```python
from build123d import *

# Parameters (mm, degrees)
SALIENTE_EXTRUIR1_DEPTH = 1.5
CROQUIS2_R              = 2.5
CROQUIS2_W              = 2.8
CROQUIS2_H              = 20
CORTAR_EXTRUIR1_DEPTH   = 11
CROQUIS4_W              = 2.8
CROQUIS4_H              = 25
CORTAR_EXTRUIR3_DEPTH   = 13
CROQUIS5_W              = 3
CROQUIS5_H              = 144.0002072
SALIENTE_EXTRUIR2_DEPTH = 15
CROQUIS6_R              = 4.1
CORTAR_EXTRUIR4_DEPTH   = 15
CROQUIS7_W              = 20.699997517
CROQUIS7_H              = 3
SALIENTE_EXTRUIR3_DEPTH = 3
CROQUIS8_W              = 20.699997553
CROQUIS8_H              = 3
SALIENTE_EXTRUIR4_DEPTH = 3


with BuildPart() as part:
    # Croquis1 → Saliente-Extruir1 (new, symmetric)
    with BuildSketch(Plane.XY):
        Polygon((419.401663173, 248.637154823), (419.401663173, 255.63715478), (422.401663173, 255.63715478), (422.401663173, 265.637154778), (419.401663173, 265.637154778), (419.401663173, 275.637154776), (422.401663173, 275.637154776), (422.401663173, 289.074445387), (426.151314195, 289.074445387), (426.151314195, 286.574445387), (429.151663171, 286.574445387), (429.151663171, 289.074445387), (431.101663171, 289.074445387), (431.101663171, 292.074445386), (429.151663171, 292.074445386), (429.151663171, 294.574864158), (426.151314195, 294.574864158), (426.151314195, 292.074445386), (422.401663173, 292.074445386), (422.401663173, 305.512154769), (419.401663173, 305.512154769), (419.401663173, 315.762154767), (422.401663173, 315.762154767), (422.401663173, 325.512154765), (419.401663173, 325.512154765), (419.401663173, 335.762154763), (422.401663173, 335.762154763), (422.401663173, 349.199445374), (426.151314195, 349.199445374), (426.151314195, 346.699445374), (429.151663171, 346.699445374), (429.151663171, 349.199445374), (431.101663171, 349.199445374), (431.101663171, 352.199445373), (429.151663171, 352.199445373), (429.151663171, 354.699864145), (426.151314195, 354.699864145), (426.151314195, 352.199445373), (422.401663173, 352.199445373), (422.401663173, 365.637154757), (419.401663173, 365.637154757), (419.401663173, 375.637154754), (422.401663173, 375.637154754), (422.401663173, 385.637154752), (419.401663173, 385.637154752), (419.401663173, 392.637154709), (431.9403463, 392.637154709), (431.9403463, 395.637154751), (444.561007671, 395.637160103), (444.561007671, 392.637160018), (453.092348422, 392.637160018), (453.092348422, 395.637160018), (462.04234842, 395.637160018), (462.04234842, 392.637192956), (464.82199969, 392.637192956), (464.82199969, 388.887541933), (462.321999691, 388.887541933), (462.321999691, 385.887192957), (464.82199969, 385.887192957), (464.82199969, 384.912192957), (467.82199969, 384.912192957), (467.82199969, 385.887192957), (470.322418461, 385.887192957), (470.322418461, 388.887541933), (467.82199969, 388.887541933), (467.82199969, 392.637192956), (470.601650959, 392.637192956), (470.601650959, 395.637192955), (479.551650957, 395.637192955), (479.551650957, 392.637269969), (488.101650956, 392.637269969), (488.101650956, 395.637269968), (500.701660095, 395.637269968), (500.701660095, 392.637258366), (519.401657648, 392.637258366), (519.401657648, 248.637051166), (500.701660131, 248.637051166), (500.701660131, 245.637039564), (488.101650991, 245.637039564), (488.101650991, 248.637039563), (479.551650993, 248.637039563), (479.551650993, 245.637116577), (470.601650995, 245.637116577), (470.601650995, 248.637116576), (467.821999725, 248.637116576), (467.821999725, 252.386767599), (470.322418497, 252.386767599), (470.322418497, 255.387116575), (467.821999725, 255.387116575), (467.821999725, 256.362116575), (464.821999726, 256.362116575), (464.821999726, 255.387116575), (462.321999727, 255.387116575), (462.321999727, 252.386767599), (464.821999726, 252.386767599), (464.821999726, 248.637116576), (462.042348456, 248.637116576), (462.042348456, 245.637149514), (453.092348458, 245.637149514), (453.092348458, 248.637149514), (444.561007707, 248.637149514), (444.561007707, 245.63714943), (431.940346335, 245.637154782), (431.940346335, 248.637154823), align=None)
    extrude(amount=SALIENTE_EXTRUIR1_DEPTH, both=True)

    # Croquis2 → Cortar-Extruir1 (cut)
    with BuildSketch(Plane.XY.offset(1.5)):
        with Locations((437.401663173, 340.137154766)):
            Circle(CROQUIS2_R)
        with Locations((437.401663173, 301.137154766)):
            Circle(CROQUIS2_R)
        with Locations((481.801663173, 320.637154766)):
            Rectangle(CROQUIS2_W, CROQUIS2_H)
        with Locations((456.001663173, 320.637154766)):
            Rectangle(CROQUIS2_W, CROQUIS2_H)
    extrude(amount=-CORTAR_EXTRUIR1_DEPTH, mode=Mode.SUBTRACT)

    # Croquis4 → Cortar-Extruir3 (cut)
    with BuildSketch(Plane(origin=(0, 0, -1.5), x_dir=(-1, 0, 0), z_dir=(0, 0, -1))):
        with Locations((-492.30166041, 320.637154766)):
            Rectangle(CROQUIS4_W, CROQUIS4_H)
    extrude(amount=-CORTAR_EXTRUIR3_DEPTH, mode=Mode.SUBTRACT)

    # Croquis5 → Saliente-Extruir2 (add)
    with BuildSketch(Plane(origin=(519.401657648, 0, 0), x_dir=(0, 0, -1), z_dir=(1, 0, 0))):
        with Locations((0, 320.637154766)):
            Rectangle(CROQUIS5_W, CROQUIS5_H)
    extrude(amount=SALIENTE_EXTRUIR2_DEPTH)

    # Croquis6 → Cortar-Extruir4 (cut)
    with BuildSketch(Plane.XY.offset(1.5)):
        with Locations((526.901657648, 257.337051166)):
            Circle(CROQUIS6_R)
        with BuildLine():
            Line((525.401657648, 369.837051166), (527.901657648, 369.837051166))
            ThreePointArc((527.901657648, 369.837051166), (528.255211039, 369.983497775), (528.401657648, 370.337051166))
            Line((528.401657648, 370.337051166), (528.401657648, 372.337051166))
            ThreePointArc((528.401657648, 372.337051166), (528.255211039, 372.690604556), (527.901657648, 372.837051166))
            Line((527.901657648, 372.837051166), (525.401657648, 372.837051166))
            Line((525.401657648, 372.837051166), (525.401657648, 369.837051166))
        make_face()
    extrude(amount=-CORTAR_EXTRUIR4_DEPTH, mode=Mode.SUBTRACT)

    # Croquis7 → Saliente-Extruir3 (add)
    with BuildSketch(Plane.XZ.offset(-248.637051166)):
        with Locations((524.05165889, 0)):
            Rectangle(CROQUIS7_W, CROQUIS7_H)
    extrude(amount=SALIENTE_EXTRUIR3_DEPTH)

    # Croquis8 → Saliente-Extruir4 (add)
    with BuildSketch(Plane(origin=(0, 392.637258366, 0), x_dir=(1, 0, 0), z_dir=(0, 1, 0))):
        with Locations((524.051658872, 0)):
            Rectangle(CROQUIS8_W, CROQUIS8_H)
    extrude(amount=SALIENTE_EXTRUIR4_DEPTH)


solid = part.part
```
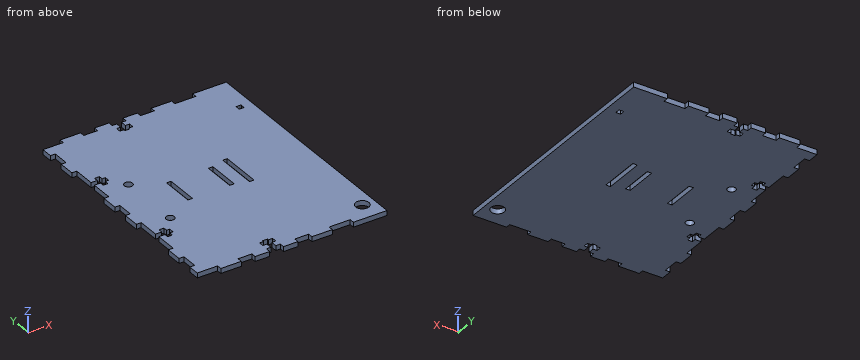
The model under review builds one solid part; all positions refer to its coordinate system, in mm. Round coordinates to 2 decimals unless told otherwise and drop trailing zeros. Loops run counter-clockwise (first coordinate to the right, second up) from the corner with the lowest first, then second, coordinate; pieces in that order, holes last. Notation, with made-up numbers: M 36.5,24 L 64.5,24 A11 cw 64.5,36 Z; hole C -22.75,1 d11. An arc over 180 degrees is marked long. Write item = value, one per line.
Item 1: Take a section at A-A on y = 323. Write out the cut boundary in (x, z), then the cut area to 3 significant figures.
Return value:
outline = M 422.4,-1.5 L 454.6,-1.5 L 454.6,1.5 L 422.4,1.5 Z; M 457.4,-1.5 L 480.4,-1.5 L 480.4,1.5 L 457.4,1.5 Z; M 483.2,-1.5 L 490.9,-1.5 L 490.9,1.5 L 483.2,1.5 Z; M 493.7,-1.5 L 534.4,-1.5 L 534.4,1.5 L 493.7,1.5 Z
area = 311 mm2
Item 2: Take a section at B-B on x = 437.5. Write out the cut boundary in (y, z).
Return value:
outline = M 245.64,-1.5 L 298.64,-1.5 L 298.64,1.5 L 245.64,1.5 Z; M 303.64,-1.5 L 337.64,-1.5 L 337.64,1.5 L 303.64,1.5 Z; M 342.64,-1.5 L 395.64,-1.5 L 395.64,1.5 L 342.64,1.5 Z
Item 3: For line 1 (X direction, y = 323, z = 0.2); line 2 (Y direction, x = 439, z = 0.3); line 3 (X direction, y = 364, z = 1.2), list the stretches that pass through material, from the lowest coordinate up. Write a range as [from, to].
Return value:
line_1 = [422.4, 454.6], [457.4, 480.4], [483.2, 490.9], [493.7, 534.4]
line_2 = [245.64, 299.21], [303.06, 338.21], [342.06, 395.64]
line_3 = [422.4, 534.4]
Item 4: Take a section at C-C on x = 450. Write out the cut boundary in (y, z).
Return value:
outline = M 248.64,-1.5 L 392.64,-1.5 L 392.64,1.5 L 248.64,1.5 Z
Item 5: Take a section at D-D on z = -0.2. State how many separate pieces and enclosed holes the cut face has, then the cut area to 3 significant figures.
Return value:
separate_pieces = 1
enclosed_holes = 7
area = 16,200 mm2
Item 6: Insertion check: P1, Ø1.5, axis at y = 324.5, z = -0.5, coming from the -X side; P2, Ø1.5, axis at x = 425, z = 0, coming from the +Y side. Each pin has a flat end and moves straight along its axis. Give the tip position at first contact, or say it passes through.
Return value:
P1 = 422.4
P2 = 392.64
